Read the model definition and answer for the solid it produces. Units are mm, in the model's axes. Face numbers are marked on the shaded views. Coordinates: 2 decimals unless noted, no trailing zeros. Order: outer loops, then holes, each group sorted by start corner. A loop starts at its lowest first (then second) coordinate and runs counter-clockwise, first axis right, second up.
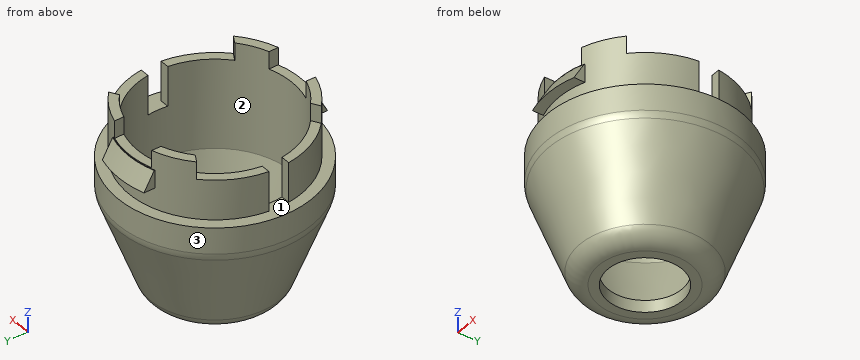
from build123d import *

# Parameters (mm, degrees)
BOX029_W               = 20
BOX029_H               = 5
BOX029_DEPTH           = 2
BOX029_PLACEMENT_ANGLE = 30
BOX027_W               = 20
BOX027_H               = 5
BOX027_DEPTH           = 2
BOX028_W               = 20
BOX028_H               = 5
BOX028_DEPTH           = 2
BOX028_PLACEMENT_ANGLE = 150
BOX030_W               = 20
BOX030_H               = 5
BOX030_DEPTH           = 2
BOX008_W               = 20
BOX008_H               = 2
BOX008_DEPTH           = 6
CYLINDER039_R          = 3.7
CYLINDER039_DEPTH      = 1.2
CYLINDER038_R          = 6
CYLINDER038_DEPTH      = 1.2
CYLINDER036_R          = 7.75
CYLINDER036_DEPTH      = 11
CYLINDER035_R          = 7.3
CYLINDER035_DEPTH      = 11
BOX007_W               = 5.6
BOX007_H               = 20
BOX007_DEPTH           = 1.8
CYLINDER037_R          = 9.75
CYLINDER037_DEPTH      = 3
CYLINDER_R             = 8.65
CYLINDER_DEPTH         = 5.75
FILLET002_R            = 2


with BuildPart() as cube029:
    # Box029 → Box029 (new body)
    with BuildSketch(Plane.XY):
        with Locations((10, 2.5)):
            Rectangle(BOX029_W, BOX029_H)
    extrude(amount=BOX029_DEPTH)


with BuildPart() as cube029_1:
    # Box029 placement: moved
    add(cube029.part.moved(Location((-7.410254, -7.165064, -1))).rotate(Axis((-7.410254, -7.165064, -1), (0, 0, 1)), BOX029_PLACEMENT_ANGLE))


with BuildPart() as cube027:
    # Box027 → Box027 (new body)
    with BuildSketch(Plane(origin=(2.5, -10, -1), x_dir=(0, 1, 0), z_dir=(0, 0, 1))):
        with Locations((10, 2.5)):
            Rectangle(BOX027_W, BOX027_H)
    extrude(amount=BOX027_DEPTH)


with BuildPart() as cube028:
    # Box028 → Box028 (new body)
    with BuildSketch(Plane.XY):
        with Locations((10, 2.5)):
            Rectangle(BOX028_W, BOX028_H)
    extrude(amount=BOX028_DEPTH)


with BuildPart() as cube028_1:
    # Box028 placement: moved
    add(cube028.part.moved(Location((9.910254, -2.834936, -1))).rotate(Axis((9.910254, -2.834936, -1), (0, 0, 1)), BOX028_PLACEMENT_ANGLE))


with BuildPart() as cube030:
    # Box030 → Box030 (new body)
    with BuildSketch(Plane(origin=(10, 2.5, -1), x_dir=(-1, 0, 0), z_dir=(0, 0, 1))):
        with Locations((10, 2.5)):
            Rectangle(BOX030_W, BOX030_H)
    extrude(amount=BOX030_DEPTH)


with BuildPart() as fusion022:
    # Box008 → Box008 (new body)
    with BuildSketch(Plane(origin=(-10, -1, -5), x_dir=(1, 0, 0), z_dir=(0, 0, 1))):
        with Locations((10, 1)):
            Rectangle(BOX008_W, BOX008_H)
    extrude(amount=BOX008_DEPTH)

    # Fusion022: union Cube029, Cube027, Cube028, Cube030
    add(cube029_1.part)
    add(cube027.part)
    add(cube028_1.part)
    add(cube030.part)


with BuildPart() as cylinder037:
    # Cylinder039 → Cylinder039 (new body)
    with BuildSketch(Plane.XY.offset(-18)):
        Circle(CYLINDER039_R)
    extrude(amount=CYLINDER039_DEPTH)


with BuildPart() as top:
    # Cylinder038 → Cylinder038 (new body)
    with BuildSketch(Plane.XY.offset(-18)):
        Circle(CYLINDER038_R)
    extrude(amount=CYLINDER038_DEPTH)

    # Cut013004: cut Cylinder037
    add(cylinder037.part, mode=Mode.SUBTRACT)


with BuildPart() as cylinder034:
    # Cylinder036 → Cylinder036 (new body)
    with BuildSketch(Plane.XY.offset(-10)):
        Circle(CYLINDER036_R)
    extrude(amount=CYLINDER036_DEPTH)


with BuildPart() as fusion015:
    # Cone003 → Cone003 (revolve)
    with BuildSketch(Plane(origin=(0, 0, -18), x_dir=(1, 0, 0), z_dir=(0, -1, 0))):
        Polygon((0, 0), (5, 0), (7.75, 8), (0, 8), align=None)
    revolve(axis=Axis((0, 0, -18), (0, 0, 1)))

    # Fusion015: union Cylinder034
    add(cylinder034.part)


with BuildPart() as cylinder033:
    # Cylinder035 → Cylinder035 (new body)
    with BuildSketch(Plane.XY.offset(-9)):
        Circle(CYLINDER035_R)
    extrude(amount=CYLINDER035_DEPTH)


with BuildPart() as cube007:
    # Box007 → Box007 (new body)
    with BuildSketch(Plane(origin=(-2.8, -10, -7.9), x_dir=(1, 0, 0), z_dir=(0, 0, 1))):
        with Locations((2.8, 10)):
            Rectangle(BOX007_W, BOX007_H)
    extrude(amount=BOX007_DEPTH)


with BuildPart() as clips:
    # Cone002 → Cone002 (revolve)
    with BuildSketch(Plane(origin=(0, 0, -8), x_dir=(1, 0, 0), z_dir=(0, -1, 0))):
        Polygon((0, 0), (9.75, 0), (8.65, 2), (0, 2), align=None)
    revolve(axis=Axis((0, 0, -8), (0, 0, 1)))

    # Common: intersect Cube007
    add(cube007.part, mode=Mode.INTERSECT)

    # Cut013002: cut Cylinder033
    add(cylinder033.part, mode=Mode.SUBTRACT)


with BuildPart() as clips_1:
    # Cut013002 placement: moved
    add(clips.part.moved(Location((0, 0, 5))))


with BuildPart() as cylinder035:
    # Cylinder037 → Cylinder037 (new body)
    with BuildSketch(Plane.XY.offset(-8)):
        Circle(CYLINDER037_R)
    extrude(amount=CYLINDER037_DEPTH)


with BuildPart() as cylinder:
    # Cylinder → Cylinder (new body)
    with BuildSketch(Plane.XY.offset(-5)):
        Circle(CYLINDER_R)
    extrude(amount=CYLINDER_DEPTH)


with BuildPart() as connector_body:
    # Cone → Cone (revolve)
    with BuildSketch(Plane(origin=(0, 0, -18), x_dir=(1, 0, 0), z_dir=(0, -1, 0))):
        Polygon((0, 0), (6, 0), (9.75, 10), (0, 10), align=None)
    revolve(axis=Axis((0, 0, -18), (0, 0, 1)))

    # Fusion014: union Clips, Cylinder035, Cylinder
    add(clips_1.part)
    add(cylinder035.part)
    add(cylinder.part)

    # Cut013003: cut Fusion015
    add(fusion015.part, mode=Mode.SUBTRACT)

    # Fusion021: union Top
    add(top.part)

    # Fillet002
    fillet002_edges = [connector_body.edges().sort_by_distance(p)[0] for p in [
        (-9.75, 0, -8),
        (-6, 0, -18),
    ]]
    fillet(fillet002_edges, radius=FILLET002_R)

    # Cut013011: cut Fusion022
    add(fusion022.part, mode=Mode.SUBTRACT)


with BuildPart() as connector_body_1:
    # Cut013011 placement: moved
    add(connector_body.part.moved(Location((0, 0, -8))))


solid = connector_body_1.part
Q1. Determine the mould class of the marked faces 1, 2 and 3 for opening direction X: +X half, -X half, draft (parallel to the pull), parting line (faces both ways), or undercut.
Q2. Straight lines are drawn through the part: L1, parallel to Y at x = 0, z = -11; L2, parallel to X at y = -6.75, z = -9.75; L3, parallel to X at y = 5, z = -15.5. For each, find the intervals that lie inside material, in ascending order.
Q3. Each of these flat-tipped pins is pushed along its axis until it touches: P1, Ø0.5, axis at y = 7.5, z = -8.5, coming from the -X side; P2, Ø4, axis at y = 4.5, z = -17, coming from the -X side; P3, Ø1, axis at x = 8, z = -10, coming from the -Y side; P4, Ø4.5, axis at x = 0, y = 0, coming from the -Z side. Where does it stop, or does it pass through?
Q4. The part is cut by section B-B, the plane z = -8.5. Determine the outline of the cut face in (x, y), then the cut area to 3 significant figures.
Computed values:
1. face 1: draft
1. face 2: undercut
1. face 3: parting line
2. L1: y = -8.65 to -7.75, 7.75 to 8.65
2. L2: x = -5.41 to -3.81, 3.81 to 5.41
2. L3: x = -8.37 to -5.92, 5.92 to 8.37
3. P1: stops at x = -4.72
3. P2: stops at x = -9.31
3. P3: stops at y = -4.31
3. P4: passes through
4. outline: (-5.92, -6.31) arc R8.65 ccw to (-2.5, -8.28) - (-2.5, -7.34) arc R7.75 cw to (-5.1, -5.83) - close; (-5.92, 6.31) - (-5.1, 5.83) arc R7.75 cw to (-2.5, 7.34) - (-2.5, 8.28) arc R8.65 ccw to start; (2.5, -8.28) arc R8.65 ccw to (5.92, -6.31) - (5.1, -5.83) arc R7.75 cw to (2.5, -7.34) - close; (2.5, 7.34) arc R7.75 cw to (5.1, 5.83) - (5.92, 6.31) arc R8.65 ccw to (2.5, 8.28) - close
4. area: 12.6 mm2
